from build123d import *

# Parameters (mm, degrees)
SKETCH8_R           = 3.5
SKETCH8_R_2         = 3
BOSS_EXTRUDE3_DEPTH = 6


with BuildPart() as part:
    # Sketch8 → Boss-Extrude3 (new body)
    with BuildSketch(Plane.XY):
        with BuildLine():
            Line((-56.665686266, -75), (-46, -75))
            Line((-46, -75), (-46, -65))
            Line((-46, -65), (-30.5, -65))
            Line((-30.5, -65), (-30.5, -57.029309822))
            Line((-30.5, -57.029309822), (-34, -57.029309822))
            Line((-34, -57.029309822), (-34, -49.029309822))
            Line((-34, -49.029309822), (-19, -49.029309822))
            Line((-19, -49.029309822), (-19, -57.029309822))
            Line((-19, -57.029309822), (-22.5, -57.029309822))
            Line((-22.5, -57.029309822), (-22.5, -65))
            Line((-22.5, -65), (22.5, -65))
            Line((22.5, -65), (22.5, -57.029309822))
            Line((22.5, -57.029309822), (19, -57.029309822))
            Line((19, -57.029309822), (19, -49.029309822))
            Line((19, -49.029309822), (34, -49.029309822))
            Line((34, -49.029309822), (34, -57.029309822))
            Line((34, -57.029309822), (30.5, -57.029309822))
            Line((30.5, -57.029309822), (30.5, -65))
            Line((30.5, -65), (46, -65))
            Line((46, -65), (46, -75))
            Line((46, -75), (56.665686266, -75))
            ThreePointArc((56.665686266, -75), (94, 0), (56.665686266, 75))
            Line((56.665686266, 75), (46, 75))
            Line((46, 75), (46, 65))
            Line((46, 65), (30.5, 65))
            Line((30.5, 65), (30.5, 57.029309822))
            Line((30.5, 57.029309822), (34, 57.029309822))
            Line((34, 57.029309822), (34, 49.029309822))
            Line((34, 49.029309822), (19, 49.029309822))
            Line((19, 49.029309822), (19, 57.029309822))
            Line((19, 57.029309822), (22.5, 57.029309822))
            Line((22.5, 57.029309822), (22.5, 65))
            Line((22.5, 65), (-22.5, 65))
            Line((-22.5, 65), (-22.5, 57.029309822))
            Line((-22.5, 57.029309822), (-19, 57.029309822))
            Line((-19, 57.029309822), (-19, 49.029309822))
            Line((-19, 49.029309822), (-34, 49.029309822))
            Line((-34, 49.029309822), (-34, 57.029309822))
            Line((-34, 57.029309822), (-30.5, 57.029309822))
            Line((-30.5, 57.029309822), (-30.5, 65))
            Line((-30.5, 65), (-46, 65))
            Line((-46, 65), (-46, 75))
            Line((-46, 75), (-56.665686266, 75))
            ThreePointArc((-56.665686266, 75), (-94, 0), (-56.665686266, -75))
        make_face()
        with Locations((-43.86, 34)):
            Circle(SKETCH8_R, mode=Mode.SUBTRACT)
        with Locations((55.5, 0)):
            Circle(SKETCH8_R, mode=Mode.SUBTRACT)
        with Locations((-43.86, -34)):
            Circle(SKETCH8_R, mode=Mode.SUBTRACT)
        Circle(SKETCH8_R_2, mode=Mode.SUBTRACT)
    extrude(amount=BOSS_EXTRUDE3_DEPTH)


solid = part.part
For this review, take the finished solid that the model builds, in its own axes (mm). A direction names the side the tool comes from. Give positions to 0.01 mm unless a question says otherwise; leave off trailing zeros. Loops run counter-clockwise (first coordinate to the right, second up) from the corner with the lowest first, then second, coordinate; pieces in that order, holes last. Notation, with made-up numbers: M 12.25,-16 L 56.25,-16 A16 cw 56.25,-1 Z; hole C -39,74 d10. An arc over 180 degrees is marked long. Put each result on its own line as item: value. Start each with the question number.
(1) Add section C-C, the plane z = 2.95. Give the number of separate pieces and of enclosed holes in the cut face, then the cut area to 3 significant figures.
(2) The part is to be moulded in two halves that separate along X. For faces 4 (the cylindrical face through (-93.992, 1.216, 2.958)), 5 (the flat face through (-1, -16, 0)), 6 (the flat face through (46, -70, 3)), say which applies: +X half, -X half, draft (parallel to the pull), parting line (faces both ways), or undercut.
(3) Add section A-A, the plane y = 0. Write out the cut boundary in (x, z), then the cut area to 3 significant figures.
(4) Add section D-D, the plane y = 34. Write out the cut boundary in (x, z).
(5) Add section B-B, the plane x = 0. Write out the cut boundary in (y, z), then the cut area to 3 significant figures.
(6) Wall thickness on L1, parallel to Y at x = -43.86, z = 2.55; L2, parallel to Y at x = -20, z = 0.55; L3, parallel to X at y = 50, z = 4.5: over which ranges is each line inside the solid? List them lowest first.
(7) For pin 1 (2 mm diameter, centred on x = -8.5, z = 2, fed in from -Y); pin 2 (1.5 mm diameter, centred on x = -19, z = 4.5, fed in from +Y); pin 3 (3 mm diameter, centred on y = -69.5, z = 2, fed in from +X); pin 4 (9 mm diameter, centred on x = -43.86, y = 34, fed in from -Z), all flat-tipped, find the tip position at first contact; note any pin that passes through.
(8) Machinability: for faces 1 (the flat face through (-22.5, 61, 3)), 2 (the flat face through (-22.5, -61, 3)), 3 (the flat face through (19, -53, 3)), which of the approach directions +Z, -Z, +X, -X, +Y, -Y give a long, thin tool a straight path to every point of the face, cutting with its end or side? Answer none if there is none.
Result:
1. separate pieces: 1
1. enclosed holes: 4
1. area: 22,100 mm^2
2. face 4: -X half
2. face 5: draft
2. face 6: undercut
3. outline: M -94,0 L -3,0 L -3,6 L -94,6 Z; M 3,0 L 52,0 L 52,6 L 3,6 Z; M 59,0 L 94,0 L 94,6 L 59,6 Z
3. area: 1,050 mm^2
4. outline: M -87.64,0 L -47.36,0 L -47.36,6 L -87.64,6 Z; M -40.36,0 L 87.64,0 L 87.64,6 L -40.36,6 Z
5. outline: M -65,0 L -3,0 L -3,6 L -65,6 Z; M 3,0 L 65,0 L 65,6 L 3,6 Z
5. area: 744 mm^2
6. L1: y = -65 to -37.5, -30.5 to 30.5, 37.5 to 65
6. L2: y = -65 to -57.03, -49.03 to 49.03, 57.03 to 65
6. L3: x = -79.6 to -34, -19 to 19, 34 to 79.6
7. pin 1: stops at y = -65
7. pin 2: stops at y = 65
7. pin 3: stops at x = 64.9
7. pin 4: stops at z = 0
8. face 1: +Z, -Z, +Y
8. face 2: +Z, -Z, -Y
8. face 3: +Z, -Z
